Could you check a few things on this model? Use its own coordinates, in mm. A direction names the side the tool comes from. Coordinates: 2 decimals unless noted, no trailing zeros. Write each loop counter-clockwise with the first axis right and the second up, starting at its lowest first coordinate (ties: lowest second). Pieces come first, ordered by that corner, then holes. Notation, with made-up numbers: (63.5, 21.25) - (84.5, 21.25) arc R21 cw to (84.5, 51.25) - close; hole circle Ø8 at (77.5, 8.5). An arc over 180 degrees is marked (long way). Answer as a JSON object with one key per item and string values. Group by question number.
1) On a 3-axis mill with a long thin cutter (end or side, diameter ignored), from which of +Z, -Z, +X, -X, +Y, -Y can I reach the whole of each face in a straight line? I mean faces 1 (the cylindrical face through (-44.423, 26.636, 0.215)), 2 (the cylindrical face through (46.65, 44.42, -0.07)), 3 (the cylindrical face through (-45.521, -41.034, 2.535)). Say none if no direction works.
2) Will these pins go through, and if not, where does the flat tip stop? pin 1 Ø2.5 at (x, y) = (24, -46.5) entering from +Z; pin 2 Ø4 at (x, y) = (-45, -45) entering from +Z; pin 3 Ø3 at (y, z) = (25, 0) entering from -X.
3) If we section it at B-B (z = -3.5): State how many separate pieces and enclosed holes the cut face has, plus the area to 3 significant figures.
4) If we section it at A-A (y = 0): Write out the boundary of the cut face in (x, z).
5) If we section it at D-D (x = 4.5): Write out the boundary of the cut face in (y, z).
6) We'd pull the mould along Y, two halves only. Please class faces 4 (the flat face through (50, 1, 0)), 5 (the conical face through (-45.286, 38.181, -0.013)), 6 (the cylindrical face through (-23.5, 0.1, -0.1)): released by +Y, released by -Y, zero draft, split by the parting line, or undercut.
7) If we section it at C-C (y = 42.5): Write out the boundary of the cut face in (x, z), plus the area to 3 significant figures.
8) Please list where these lines run through material, in increasing order: line 1 along Y through (x, z) = (0, 1); line 2 along Y through (x, z) = (25, 2.9); line 3 along X through (y, z) = (-6, -2.5).
```python
from build123d import *

# Parameters (mm, degrees)
SKETCH1_W                                           = 10
SKETCH1_H                                           = 100
BOSS_EXTRUDE1_DEPTH                                 = 50
SKETCH2_R                                           = 15
CUT_EXTRUDE1_DEPTH                                  = 10
CBORE_FOR_M4_HEX_SOCKET_HEAD_CAP_SCREW1_D           = 4.5
CBORE_FOR_M4_HEX_SOCKET_HEAD_CAP_SCREW1_CBORE_D     = 8
CBORE_FOR_M4_HEX_SOCKET_HEAD_CAP_SCREW1_CBORE_DEPTH = 5
M4_TAPPED_HOLE1_D                                   = 3.3
M4_TAPPED_HOLE1_DEPTH                               = 11
M4_TAPPED_HOLE1_TIP                                 = 0.991420021
M4_TAPPED_HOLE2_D                                   = 3.3
M4_TAPPED_HOLE2_DEPTH                               = 11
M4_TAPPED_HOLE2_TIP                                 = 0.991420021
M4_TAPPED_HOLE3_D                                   = 3.3
M4_TAPPED_HOLE3_DEPTH                               = 11
M4_TAPPED_HOLE3_TIP                                 = 0.991420021
M6_TAPPED_HOLE1_D                                   = 5


with BuildPart() as part:
    # Sketch1 → Boss-Extrude1 (new, symmetric)
    with BuildSketch(Plane(origin=(0, 0, 0), x_dir=(0, 0, -1), z_dir=(1, 0, 0))):
        Rectangle(SKETCH1_W, SKETCH1_H)
    extrude(amount=BOSS_EXTRUDE1_DEPTH, both=True)

    # Sketch2 → Cut-Extrude1 (cut)
    with BuildSketch(Plane.XY.offset(5)):
        Circle(SKETCH2_R)
    extrude(amount=-CUT_EXTRUDE1_DEPTH, mode=Mode.SUBTRACT)

    # CBORE for M4 Hex Socket Head Cap Screw1 (through all)
    with Locations(Plane.XY.offset(5)):
        with Locations((-45, -45), (-25, -45), (25, -45), (45, -45)):
            CounterBoreHole(CBORE_FOR_M4_HEX_SOCKET_HEAD_CAP_SCREW1_D / 2, CBORE_FOR_M4_HEX_SOCKET_HEAD_CAP_SCREW1_CBORE_D / 2, CBORE_FOR_M4_HEX_SOCKET_HEAD_CAP_SCREW1_CBORE_DEPTH)

    # M4 Tapped Hole1
    with Locations(Plane(origin=(0, 50, 0), x_dir=(1, 0, 0), z_dir=(0, 1, 0))):
        with Locations((-45, 0), (-25, 0), (25, 0), (45, 0)):
            Hole(M4_TAPPED_HOLE1_D / 2, depth=M4_TAPPED_HOLE1_DEPTH)
            with Locations((0, 0, -(M4_TAPPED_HOLE1_DEPTH + M4_TAPPED_HOLE1_TIP / 2))):  # 118° drill point
                Cone(0, M4_TAPPED_HOLE1_D / 2, M4_TAPPED_HOLE1_TIP, mode=Mode.SUBTRACT)

    # M4 Tapped Hole2
    with Locations(Plane.ZY.offset(50)):
        with Locations((0, 25), (0, -25)):
            Hole(M4_TAPPED_HOLE2_D / 2, depth=M4_TAPPED_HOLE2_DEPTH)
            with Locations((0, 0, -(M4_TAPPED_HOLE2_DEPTH + M4_TAPPED_HOLE2_TIP / 2))):  # 118° drill point
                Cone(0, M4_TAPPED_HOLE2_D / 2, M4_TAPPED_HOLE2_TIP, mode=Mode.SUBTRACT)

    # M4 Tapped Hole3
    with Locations(Plane(origin=(50, 0, 0), x_dir=(0, 0, -1), z_dir=(1, 0, 0))):
        with Locations((0, 25), (0, -25)):
            Hole(M4_TAPPED_HOLE3_D / 2, depth=M4_TAPPED_HOLE3_DEPTH)
            with Locations((0, 0, -(M4_TAPPED_HOLE3_DEPTH + M4_TAPPED_HOLE3_TIP / 2))):  # 118° drill point
                Cone(0, M4_TAPPED_HOLE3_D / 2, M4_TAPPED_HOLE3_TIP, mode=Mode.SUBTRACT)

    # M6 Tapped Hole1 (through all)
    with Locations(Plane.XY.offset(5)):
        with Locations((0, 26), (-26, 0), (26, 0), (0, -26)):
            Hole(M6_TAPPED_HOLE1_D / 2)


solid = part.part
```
Here are the results:
{
 "1": {"face 1": "-X", "face 2": "+Y", "face 3": "+Z"},
 "2": {"pin 1": "stops at z = 0", "pin 2": "passes through", "pin 3": "stops at x = -38.91"},
 "3": {"separate pieces": "1", "enclosed holes": "9", "area": "9,150 mm²"},
 "4": {"outline": "(-50, -5) - (-28.5, -5) - (-28.5, 5) - (-50, 5) - close; (-23.5, -5) - (-15, -5) - (-15, 5) - (-23.5, 5) - close; (15, -5) - (23.5, -5) - (23.5, 5) - (15, 5) - close; (28.5, -5) - (50, -5) - (50, 5) - (28.5, 5) - close"},
 "5": {"outline": "(-50, -5) - (-14.31, -5) - (-14.31, 5) - (-50, 5) - close; (14.31, -5) - (50, -5) - (50, 5) - (14.31, 5) - close"},
 "6": {"face 4": "zero draft", "face 5": "released by +Y", "face 6": "undercut"},
 "7": {"outline": "(-50, -5) - (50, -5) - (50, 5) - (-50, 5) - close; hole circle Ø3.3 at (-45, 0); hole circle Ø3.3 at (-25, 0); hole circle Ø3.3 at (25, 0); hole circle Ø3.3 at (45, 0)", "area": "966 mm²"},
 "8": {"line 1": "y = -50 to -28.5, -23.5 to -15, 15 to 23.5, 28.5 to 50", "line 2": "y = -50 to -49, -41 to -2.29, 2.29 to 50", "line 3": "x = -50 to -13.75, 13.75 to 50"}
}
